from build123d import *

# Parameters (mm, degrees)
ESBO_O1_R                = 4
ESBO_O1_W                = 11
ESBO_O1_H                = 5
RESSALTO_EXTRUS_O1_DEPTH = 13
RESSALTO_EXTRUS_O3_START = -36
RESSALTO_EXTRUS_O3_DEPTH = 10
CORTE_EXTRUS_O2_START    = -10
ESBO_O7_R                = 8
CORTE_EXTRUS_O2_DEPTH    = 2.3
CORTE_EXTRUS_O3_START    = -2.3
ESBO_O7_2_R              = 8
CORTE_EXTRUS_O3_DEPTH    = 2.3
ESBO_O8_W                = 5.6
ESBO_O8_H                = 2.5
CORTE_EXTRUS_O4_DEPTH    = 10
ESBO_O9_R                = 1.75
CORTE_EXTRUS_O5_DEPTH    = 90.578178146


with BuildPart() as part:
    # Esbo_o1 → Ressalto-extrus_o1 (new body)
    with BuildSketch(Plane.XY):
        with BuildLine():
            Line((4, 6.34428877), (4, 63.65571123))
            ThreePointArc((4, 63.65571123), (6.704091727, 73.362313803), (-2.692582404, 77))
            Line((-2.692582404, 77), (-19, 77))
            Line((-19, 77), (-19, 53))
            Line((-19, 53), (-19, 41))
            Line((-19, 41), (-4, 41))
            Line((-4, 41), (-4, 6.34428877))
            ThreePointArc((-4, 6.34428877), (0, -7.5), (4, 6.34428877))
        make_face()
        Circle(ESBO_O1_R, mode=Mode.SUBTRACT)
        with Locations((-9.5, 47.5)):
            Rectangle(ESBO_O1_W, ESBO_O1_H, mode=Mode.SUBTRACT)
        with Locations((0, 70)):
            Circle(ESBO_O1_R, mode=Mode.SUBTRACT)
    extrude(amount=RESSALTO_EXTRUS_O1_DEPTH)

    # Esbo_o5 → Ressalto-extrus_o3 (add)
    with BuildSketch(Plane.XZ.offset(-41).offset(RESSALTO_EXTRUS_O3_START)):
        with BuildLine():
            Line((-21, 13), (-19, 13))
            Line((-19, 13), (-19, 0))
            Line((-19, 0), (-43, 0))
            Line((-43, 0), (-43, 13))
            Line((-43, 13), (-35.5, 13))
            ThreePointArc((-35.5, 13), (-30, 7.5), (-24.5, 13))
            Line((-24.5, 13), (-21, 13))
        make_face()
    extrude(amount=RESSALTO_EXTRUS_O3_DEPTH)

    # Esbo_o7 → Corte-extrus_o2 (cut)
    with BuildSketch(Plane(origin=(0, 77, 0), x_dir=(1, 0, 0), z_dir=(0, 1, 0)).offset(CORTE_EXTRUS_O2_START)):
        with Locations((-30, -13)):
            Circle(ESBO_O7_R)
    extrude(amount=CORTE_EXTRUS_O2_DEPTH, mode=Mode.SUBTRACT)

    # Esbo_o7_2 → Corte-extrus_o3 (cut)
    with BuildSketch(Plane(origin=(0, 77, 0), x_dir=(1, 0, 0), z_dir=(0, 1, 0)).offset(CORTE_EXTRUS_O3_START)):
        with Locations((-30, -13)):
            Circle(ESBO_O7_2_R)
    extrude(amount=CORTE_EXTRUS_O3_DEPTH, mode=Mode.SUBTRACT)

    # Esbo_o8 → Corte-extrus_o4 (cut)
    with BuildSketch(Plane(origin=(0, 77, 0), x_dir=(1, 0, 0), z_dir=(0, 1, 0))):
        with Locations((-38, -4)):
            Rectangle(ESBO_O8_W, ESBO_O8_H)
        with Locations((-22, -4)):
            Rectangle(ESBO_O8_W, ESBO_O8_H)
    extrude(amount=-CORTE_EXTRUS_O4_DEPTH, mode=Mode.SUBTRACT)

    # Esbo_o9 → Corte-extrus_o5 (cut, through all)
    with BuildSketch(Plane.XY.offset(13)):
        with Locations((-38, 72)):
            Circle(ESBO_O9_R)
        with Locations((-22, 72)):
            Circle(ESBO_O9_R)
    extrude(amount=-CORTE_EXTRUS_O5_DEPTH, mode=Mode.SUBTRACT)


solid = part.part
Input: part model. Units: mm. Frame: model coordinates. A direction names the side the tool comes from. Coordinates: 2 decimals unless noted, no trailing zeros. Loops run counter-clockwise (first coordinate to the right, second up) from the corner with the lowest first, then second, coordinate; pieces in that order, holes last.
Q1. Cut plane C-C (x = -13). Output: boundary loops of the cut face in (y, z), then the cut area to 3 significant figures.
Q2. Set-up query: faces 1 (the face through (-12, 41, 6)), 2 (the face through (-18, 77, 7)), 3 (the face through (-30, 69.3, 7)), 4 (the face through (-40, 72, 2.75)). Return all of +Z, -Z, +X, -X, +Y, -Y with unobstructed straight access to the full face (end or side cutting, diameter ignored); none if empty.
Q3. Cut plane A-A (z = 3.75). Output: boundary loops of the cut face in (x, y).
Q4. Draft query along Y for faces 5 (the face through (4, 35, 6)), 6 (the face through (-31, 67, 4)), 7 (the face through (-15, 47, 6)), 8 (the face through (-30, 76, 5)). Return one class per face: +Y half, -Y half, draft (parallel to the pull), parting line (faces both ways), or undercut.
Q5. Contact query for flat-ended pins moving along their axis: pin 1 (5 mm diameter, centred on x = -21.5, z = 11.5, fed in from +Y); pin 2 (12 mm diameter, centred on x = -22, y = 34, fed in from +Z); pin 3 (4 mm diameter, centred on y = 34.5, z = 6, fed in from +X); pin 4 (6 mm diameter, centred on x = -19.5, z = 6, fed in from -Y). Output: stop coordinate, or through.
Q6. Cut plane D-D (x = 0). Output: boundary loops of the cut face in (y, z), then the cut area to 3 significant figures.
Q7. Cut plane B-B (y = 48). Output: boundary loops of the cut face in (x, z).
Q8. Material intervals for line 1 (X direction, y = 34, z = 3.25); line 2 (Y direction, x = -38, z = 7.5); line 3 (X direction, y = 72, z = 7), sorted ascending.
Working result:
1. outline: (41, 0) - (45, 0) - (45, 13) - (41, 13) - close; (50, 0) - (77, 0) - (77, 13) - (50, 13) - close
1. area: 403 mm2
2. face 1: +Z, -Z, -X
2. face 2: +Z, -Z, -X, +Y
2. face 3: +Z, -Y
2. face 4: +Y, -Y
3. outline: (-43, 67) - (-40.8, 67) - (-40.8, 77) - (-43, 77) - close; (-35.2, 67) - (-24.8, 67) - (-24.8, 77) - (-35.2, 77) - close; (-19.2, 67) - (-19, 67) - (-19, 41) - (-4, 41) - (-4, 6.34) arc R7.5 ccw (long way) to (4, 6.34) - (4, 63.66) arc R7.5 ccw to (-2.69, 77) - (-19.2, 77) - close; hole (-15, 45) - (-4, 45) - (-4, 50) - (-15, 50) - close; hole circle Ø8 at (0, 0); hole circle Ø8 at (0, 70)
4. face 5: undercut
4. face 6: -Y half
4. face 7: undercut
4. face 8: draft
5. pin 1: stops at y = 77
5. pin 2: passes through
5. pin 3: stops at x = 4
5. pin 4: stops at y = 41
6. outline: (-7.5, 0) - (-4, 0) - (-4, 13) - (-7.5, 13) - close; (4, 0) - (66, 0) - (66, 13) - (4, 13) - close; (74, 0) - (77.5, 0) - (77.5, 13) - (74, 13) - close
6. area: 897 mm2
7. outline: (-19, 0) - (-15, 0) - (-15, 13) - (-19, 13) - close; (-4, 0) - (4, 0) - (4, 13) - (-4, 13) - close
8. line 1: x = -4 to 4
8. line 2: y = 67 to 70.25, 73.75 to 77
8. line 3: x = -43 to -39.75, -36.25 to -23.75, -20.25 to -3.46, 3.46 to 7.23
